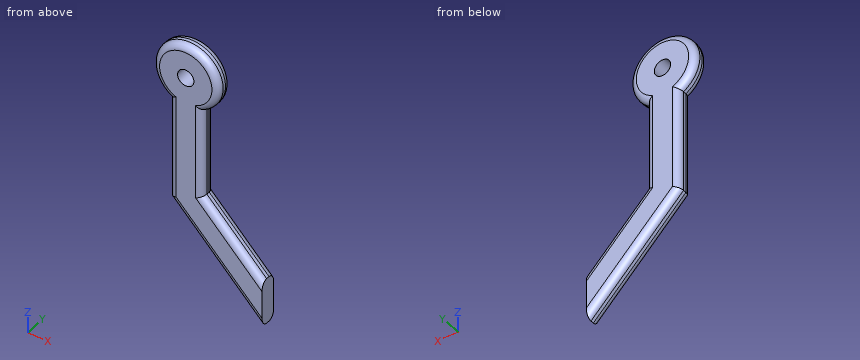
Autodesk Inventor part; units mm, degrees
ref_plane "YZ Plane" through (0, 0, 0) normal (1, 0, 0) x (0, 1, 0)
ref_plane "XZ Plane" through (0, 0, 0) normal (0, 1, 0) x (-1, 0, 0)
ref_plane "XY Plane" through (0, 0, 0) normal (0, 0, 1) x (1, 0, 0)
sketch "Sketch1" plane through (0, 0, 0) normal (0, 1, 0) x (-1, 0, 0)
  line L0 (5, -20) -> (5, 11.3397)
  line L1 (-5, 11.3397) -> (-5, -15.8579)
  arc A0 (5, 11.3397) -> (-5, 11.3397) centre (0, 20) ccw
  line L2 (5, -20) -> (-23.2843, -48.2843)
  line L3 (-23.2843, -34.1421) -> (-5, -15.8579)
  line L4 (5, -20) -> (45, -20) construction
  line L5 (-23.2843, -48.2843) -> (-23.2843, -34.1421)
  circle A1 centre (0, 20) radius 2.5
  point P0 (0, 0)
  dimension "d2" = 20
  dimension "d8" = 135
  dimension "d14" = 23.2843
extrude "Extrusion1" add sketch "Sketch1" along normal blind 5
fillet "Fillet1" radius 2 10 edges at (0, 5, 30) (0, 0, 30) (5, 5, -2.2591) (-5, 5, -4.3301) (5, 0, -2.2591) (-5, 0, -4.3301) (9.1421, 0, -34.1421) (9.1421, 5, -34.1421) (14.1421, 0, -25) (14.1421, 5, -25)
properties part number "Gripper"
Build history of the part. All positions in model axes, mm. Coordinates: 2 decimals unless noted, no trailing zeros. Order: outer loops, then holes, each group sorted by start corner. A loop starts at its lowest first (then second) coordinate and runs counter-clockwise, first axis right, second up. Notation, with made-up numbers: (49.5, 22) - (87.5, 22) arc R12 cw to (87.5, 33) - close; hole circle Ø4 at (-24.75, -12). An arc over 180 degrees is marked (long way). Put each result on its own line as item: value.
1. Drop flat-ended pins along their axis: P1, Ø1.5, axis at x = -6, y = 2.5, coming from the -Z side; P2, Ø0.8, axis at y = 2.5, z = 1.5, coming from the +X side. Give the stop position or say it passes through.
Answer sheet:
P1: stops at z = 11.49
P2: stops at x = 5
2. Saw through at A-A (y = 3.85). Write the cut outline in (x, z), and give its area (3 significant figures).
Answer sheet:
outline: (-4.81, -19.92) - (23.28, -48.02) - (23.28, -34.41) - (4.81, -15.94) - (4.81, 11.45) arc R9.81 ccw (long way) to (-4.81, 11.45) - close; hole circle Ø5 at (0, 20)
area: 874 mm^2
3. Saw through at B-B (z = 20). Write the cut outline in (x, y), and give its area (3 significant figures).
Answer sheet:
outline: (-10, 2) arc R2 ccw to (-8, 0) - (-2.5, 0) - (-2.5, 5) - (-8, 5) arc R2 ccw to (-10, 3) - close; (2.5, 0) - (8, 0) arc R2 ccw to (10, 2) - (10, 3) arc R2 ccw to (8, 5) - (2.5, 5) - close
area: 71.6 mm^2
4. Probe line 1 along Z through (x, y) = (8, 4.3); line 2 along Z through (x, y) = (0.5, 2); line 3 along X through (y, z) = (4.1, 24). List the from-to ranges inside material, lowest first. Write a range as [from, to].
Answer sheet:
line 1: z = [-32.32, -19.54], [14.84, 25.16]
line 2: z = [-25.5, 17.55], [22.45, 29.99]
line 3: x = [-8.8, 8.8]
